Verification items for the finished model (mm, model axes). A direction names the side the tool comes from. Give positions to 0.01 mm unless a question says otherwise; leave off trailing zeros. Loops run counter-clockwise (first coordinate to the right, second up) from the corner with the lowest first, then second, coordinate; pieces in that order, holes last. Notation, with made-up numbers: M -27.75,85 L -17.75,85 A24 ccw -17.75,104 Z; hole C -12,68 d2. An arc over 180 degrees is marked long. Answer in a Markdown table with one row per item.
```python
from build123d import *

# Parameters (mm, degrees)
SKETCH1_W           = 154
SKETCH1_H           = 154
SKETCH1_W_2         = 150
SKETCH1_H_2         = 150
BOSS_EXTRUDE1_DEPTH = 250
SKETCH2_W           = 154
SKETCH2_H           = 154
SKETCH2_R           = 20
SKETCH2_R_2         = 4
BOSS_EXTRUDE2_DEPTH = 2
BOSS_EXTRUDE3_DEPTH = 50
SKETCH4_W           = 49
SKETCH4_H           = 49
BOSS_EXTRUDE4_DEPTH = 2
SKETCH5_W           = 4
SKETCH5_H           = 45
CUT_EXTRUDE1_DEPTH  = 2
SKETCH6_R           = 4
CUT_EXTRUDE2_DEPTH  = 70
SKETCH9_R           = 74
SKETCH9_R_2         = 72
BOSS_EXTRUDE9_DEPTH = 50


with BuildPart() as part:
    # Sketch1 → Boss-Extrude1 (new body)
    with BuildSketch(Plane.XY):
        Rectangle(SKETCH1_W, SKETCH1_H)
        Rectangle(SKETCH1_W_2, SKETCH1_H_2, mode=Mode.SUBTRACT)
    extrude(amount=BOSS_EXTRUDE1_DEPTH)

    # Sketch2 → Boss-Extrude2 (add)
    with BuildSketch(Plane(origin=(0, 0, 0), x_dir=(-1, 0, 0), z_dir=(0, 0, -1))):
        Rectangle(SKETCH2_W, SKETCH2_H)
        with Locations((0, 40)):
            Circle(SKETCH2_R, mode=Mode.SUBTRACT)
        Circle(SKETCH2_R_2, mode=Mode.SUBTRACT)
    extrude(amount=BOSS_EXTRUDE2_DEPTH)

    # Sketch3 → Boss-Extrude3 (add)
    with BuildSketch(Plane(origin=(0, 0, -2), x_dir=(-1, 0, 0), z_dir=(0, 0, -1))):
        Polygon((2, 64.5), (2, 62.5), (0, 62.5), (-22.5, 62.5), (-22.5, 17.5), (0, 17.5), (2, 17.5), (2, 15.5), (-24.5, 15.5), (-24.5, 64.5), align=None)
    extrude(amount=BOSS_EXTRUDE3_DEPTH)

    # Sketch4 → Boss-Extrude4 (add)
    with BuildSketch(Plane(origin=(0, 0, -52), x_dir=(-1, 0, 0), z_dir=(0, 0, -1))):
        with Locations((0, 40)):
            Rectangle(SKETCH4_W, SKETCH4_H)
    extrude(amount=BOSS_EXTRUDE4_DEPTH)

    # Sketch5 → Cut-Extrude1 (cut)
    with BuildSketch(Plane(origin=(24.5, 0, 0), x_dir=(0, 0, -1), z_dir=(1, 0, 0))):
        with Locations((4, 40)):
            Rectangle(SKETCH5_W, SKETCH5_H)
    extrude(amount=-CUT_EXTRUDE1_DEPTH, mode=Mode.SUBTRACT)

    # Sketch6 → Cut-Extrude2 (cut)
    with BuildSketch(Plane(origin=(24.5, 0, 0), x_dir=(0, 0, -1), z_dir=(1, 0, 0))):
        with Locations((32, 40)):
            Circle(SKETCH6_R)
    extrude(amount=-CUT_EXTRUDE2_DEPTH, mode=Mode.SUBTRACT)

    # Sketch9 → Boss-Extrude9 (add)
    with BuildSketch(Plane.XY):
        with Locations(Location((0, 0, 0), (0, 0, 180))):
            Circle(SKETCH9_R)
        Circle(SKETCH9_R_2, mode=Mode.SUBTRACT)
    extrude(amount=BOSS_EXTRUDE9_DEPTH)


solid = part.part
```
Item 1: Scan lines: L1, parallel to X at y = 65.5, z = 81.5; L2, parallel to Y at x = 23.35, z = -32; L3, parallel to X at y = -10, z = 32.5. Record each from-to range of solid material in increasing order. Write a range as [from, to].
Reported:
| item | result |
|---|---|
| L1 | x = [-77, -75], [75, 77] |
| L2 | y = [15.5, 36], [44, 64.5] |
| L3 | x = [-77, -75], [-73.32, -71.3], [71.3, 73.32], [75, 77] |
Item 2: Sectioned sample at A-A (z = 18.5). Record the cut outline in (x, y), and give its area (3 significant figures).
Reported:
| item | result |
|---|---|
| outline | M -77,-77 L 77,-77 L 77,77 L -77,77 Z; C 0,0 d148; hole M -75,-75 L 75,-75 L 75,75 L -75,75 Z; hole C 0,0 d144 |
| area | 2,130 mm^2 |
Item 3: Sectioned sample at B-B (y = 0). Record the cut outline in (x, z), and give its area (3 significant figures).
Reported:
| item | result |
|---|---|
| outline | M -77,-2 L -4,-2 L -4,0 L -72,0 L -72,50 L -74,50 L -74,0 L -75,0 L -75,250 L -77,250 Z; M 4,-2 L 77,-2 L 77,250 L 75,250 L 75,0 L 74,0 L 74,50 L 72,50 L 72,0 L 4,0 Z |
| area | 1,490 mm^2 |
Item 4: Sectioned sample at D-D (y = 40). State how many separate pieces and enclosed holes the cut face has, and give its area (3 significant figures).
Reported:
| item | result |
|---|---|
| separate pieces | 4 |
| enclosed holes | 0 |
| area | 1,640 mm^2 |
Item 5: Tool access check on faces 1 (the flat face through (11, 64.5, -28)), 2 (the flat face through (75, -1, 123)), 3 (the flat face through (-1, 40, -52)). Record the directions out of +Z, -Z, +X, -X, +Y, -Y that give a thin tool (end or side, any length) a straight path to the whole face; none if there is none.
Reported:
| item | result |
|---|---|
| face 1 | -Z, +X, -X, +Y |
| face 2 | +Z |
| face 3 | -X |
Item 6: Go/stop test with flat-tipped pins: pin 1 (12 mm diameter, centred on x = -13.5, y = 24, fed in from +Z); pin 2 (14.5 mm diameter, centred on x = 6.5, z = -29.5, fed in from +Y); pin 3 (24.5 mm diameter, centred on x = -8.5, z = -19.5, fed in from -Y). Record where each tip stops, or that it passes through.
Reported:
| item | result |
|---|---|
| pin 1 | stops at z = 0 |
| pin 2 | stops at y = 64.5 |
| pin 3 | stops at y = 15.5 |
Item 7: Sectioned sample at C-C (z = 219). Record the cut outline in (x, y).
Reported:
| item | result |
|---|---|
| outline | M -77,-77 L 77,-77 L 77,77 L -77,77 Z; hole M -75,-75 L 75,-75 L 75,75 L -75,75 Z |
Item 8: Release check for a two-part mould opening along Z. For faces 4 (the flat face through (0, 40, -54)), 5 (the cylindrical face through (23.514, 43.966, -31.479)), 6 (the flat face through (1, -77, 126)) record: released by +Z, released by -Z, zero draft, split by the parting line, or undercut.
Reported:
| item | result |
|---|---|
| face 4 | released by -Z |
| face 5 | undercut |
| face 6 | zero draft |
